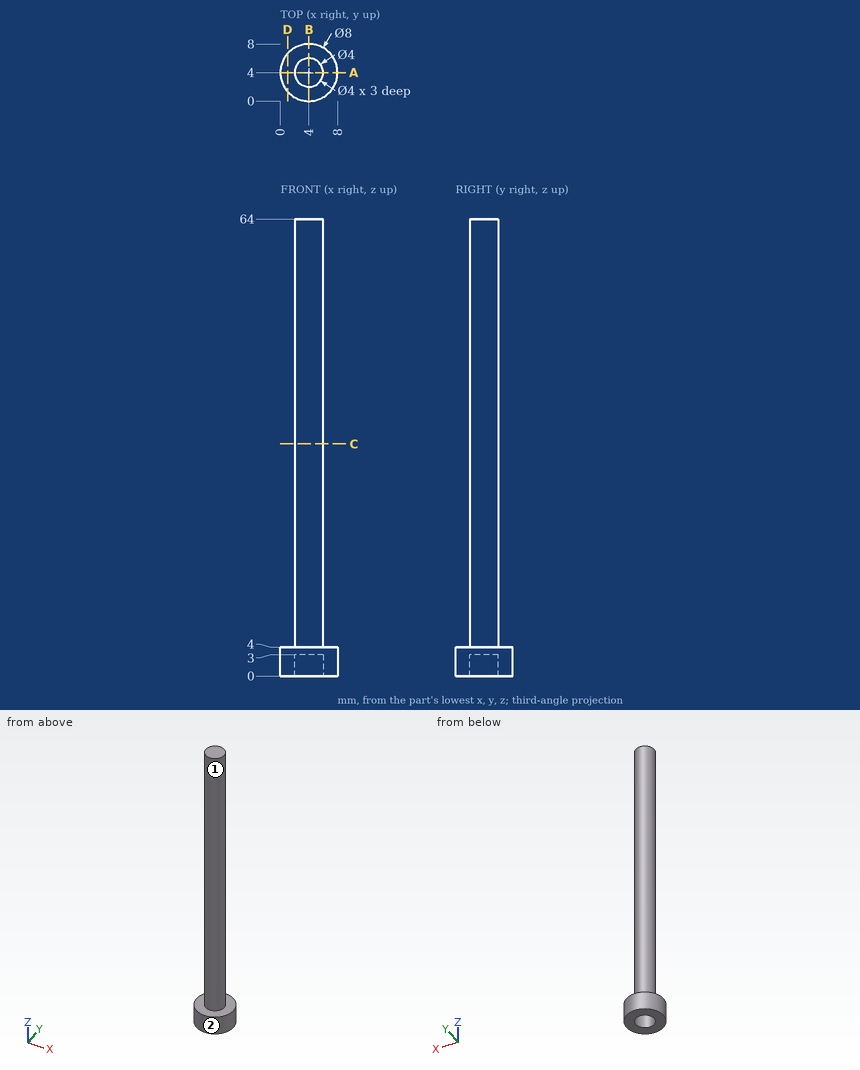
Input: dimensioned drawing with shaded views. Units: mm. Origin: part minimum x, y, z. A direction names the side the tool comes from. Round coordinates to 2 decimals unless told otherwise and drop trailing zeros. Order: outer loops, then holes, each group sorted by start corner. A loop starts at its lowest first (then second) coordinate and runs counter-clockwise, first axis right, second up.
Q1. Section A-A, the plane y = 4. Output: boundary loops of the cut face in (x, z), and give its area (3 significant figures).
Result sheet:
outline: (0, 0) - (2, 0) - (2, 3) - (6, 3) - (6, 0) - (8, 0) - (8, 4) - (6, 4) - (6, 64) - (2, 64) - (2, 4) - (0, 4) - close
area: 260 mm2
Q2. Access query for the marked faces 1 and 2. Directions: +Z, -Z, +X, -X, +Y, -Y. A direction counts if a zero-diameter tool reaches every point of the face in a straight line with its end or side. Return the directions, or none.
Result sheet:
face 1: +Z
face 2: +Z, -Z
Q3. Section D-D, the plane x = 1. Output: boundary loops of the cut face in (y, z), and give its area (3 significant figures).
Result sheet:
outline: (1.35, 0) - (6.65, 0) - (6.65, 4) - (1.35, 4) - close
area: 21.2 mm2
Q4. Section C-C, the plane z = 32.5. Output: boundary loops of the cut face in (x, y).
Result sheet:
outline: circle Ø4 at (4, 4)
Q5. Pin query (flat end, axial travel): pin 1 (1.5 mm diameter, centred on x = 2, y = 2, fed in from +Z); pin 2 (4 mm diameter, centred on x = 6, z = 8, fed in from -Y); pin 3 (1.5 mm diameter, centred on y = 3.5, z = 25.5, fed in from +X). Return the tip coordinate at first contact, or that it passes through.
Result sheet:
pin 1: stops at z = 4
pin 2: stops at y = 2
pin 3: stops at x = 6
Q6. Material intervals for probe 1 along Y at (x, z) = (4, 1.5); probe 2 along Z at (x, y) = (1.5, 3.75); probe 3 along Z at (x, y) = (4.75, 2.25), sorted ascending.
Result sheet:
probe 1: y = 0 to 2, 6 to 8
probe 2: z = 0 to 4
probe 3: z = 3 to 64
